The listing builds one solid part. Answer for the finished solid, in the listing's coordinates (mm). A direction names the side the tool comes from. Give positions to 0.01 mm unless a question says otherwise; leave off trailing zeros. Loops run counter-clockwise (first coordinate to the right, second up) from the corner with the lowest first, then second, coordinate; pieces in that order, holes last. Notation, with made-up numbers: M 13.5,-24 L 36.5,-24 A28 ccw 36.5,15 Z; hole C -3.5,-13.75 d8. An arc over 180 degrees is marked long. Return JSON: item names as keys, results as strings.
from build123d import *

# Parameters (mm, degrees)
SKETCH_1_W          = 54.664318292
SKETCH_1_H          = 5
SKETCH_1_R          = 1.5
EXTRUDE_1_DEPTH     = 5
SKETCH_2_W          = 59.460193076
SKETCH_2_H          = 2.500348526
EXTRUDE_2_DEPTH     = 23
SKETCH_5_R          = 16.5
CUT_EXTRUDE_1_DEPTH = 15
EXTRUDE_START       = 5
EXTRUDE_3_DEPTH     = 5
CHAMFER_1_SIZE      = 5
FILLET_6_R          = 10
FILLET_7_R          = 4
FILLET_8_R          = 5
FILLET_9_R          = 3


with BuildPart() as part:
    # 草图1 → 凸台-拉伸1 (new body)
    with BuildSketch(Plane(origin=(0, 0, 0), x_dir=(1, 0, 0), z_dir=(0, 1, 0))):
        with Locations((1.075531559, -8.61)):
            Rectangle(SKETCH_1_W, SKETCH_1_H)
        with Locations(Location((-10, -8.5, 0), (0, 0, 270))):
            Circle(SKETCH_1_R, mode=Mode.SUBTRACT)
        with Locations(Location((10, -8.5, 0), (0, 0, 90))):
            Circle(SKETCH_1_R, mode=Mode.SUBTRACT)
    extrude(amount=EXTRUDE_1_DEPTH)

    # 草图2 → 凸台-拉伸2 (add)
    with BuildSketch(Plane.XY.offset(11.11)):
        with Locations((0, 2.5)):
            Rectangle(SKETCH_2_W, SKETCH_2_H)
    extrude(amount=EXTRUDE_2_DEPTH)

    # 草图5 → 切除-拉伸1 (cut)
    with BuildSketch(Plane(origin=(0, 3.750174263, 0), x_dir=(1, 0, 0), z_dir=(0, 1, 0))):
        with Locations((-0.32, -44.994124541)):
            Circle(SKETCH_5_R)
    extrude(amount=-CUT_EXTRUDE_1_DEPTH, mode=Mode.SUBTRACT)

    # 草图7 → 凸台-拉伸3 (add)
    with BuildSketch(Plane(origin=(0, 3.750174263, 0), x_dir=(1, 0, 0), z_dir=(0, 1, 0)).offset(EXTRUDE_START)):
        with BuildLine():
            Line((29.730096538, -11.11), (28.407690705, -11.11))
            Line((28.407690705, -11.11), (-26.256627587, -11.11))
            Line((-26.256627587, -11.11), (-29.730096538, -11.11))
            Line((-29.730096538, -11.11), (-29.730096538, -34.11))
            Line((-29.730096538, -34.11), (-12.721041608, -34.11))
            ThreePointArc((-12.721041608, -34.11), (-0.32, -28.494124541), (12.081041608, -34.11))
            Line((12.081041608, -34.11), (29.730096538, -34.11))
            Line((29.730096538, -34.11), (29.730096538, -11.11))
        make_face()
    extrude(amount=-EXTRUDE_3_DEPTH)

    # 倒角1
    # the kernel refuses this chamfer: 5 mm, written as the material it takes off along each edge
    with BuildSketch(Plane(origin=(-42.588511478, 8.750174263, 11.11), x_dir=(0, -0.9996219169112968, -0.027495876610586317), z_dir=(1, 0, 0))) as chamfer_1_piece_1_section:
        Polygon((CHAMFER_1_SIZE * 0.999621916911, -CHAMFER_1_SIZE * 0.0274958766106), (-CHAMFER_1_SIZE * 0.0274958766106, -CHAMFER_1_SIZE * 0.999621916911), (0, 0), align=None)
    chamfer_1_piece_1 = extrude(amount=85.177022955, mode=Mode.PRIVATE)
    chamfer_1_piece_1 = split(chamfer_1_piece_1, bisect_by=Plane(origin=(-34.422569532, 5, 11.399404242), z_dir=(0, -1, 0)), keep=Keep.TOP, mode=Mode.PRIVATE)
    chamfer_1_piece_1 = split(chamfer_1_piece_1, bisect_by=Plane(origin=(-26.256627587, 4.506210637, 11.399404242), z_dir=(-1, 0, 0)), keep=Keep.TOP, mode=Mode.PRIVATE)
    add(chamfer_1_piece_1, mode=Mode.SUBTRACT)
    with BuildSketch(Plane(origin=(-42.588511478, 8.750174263, 11.11), x_dir=(0, -0.9996219169112968, -0.027495876610586317), z_dir=(1, 0, 0))) as chamfer_1_piece_2_section:
        Polygon((CHAMFER_1_SIZE * 0.999621916911, -CHAMFER_1_SIZE * 0.0274958766106), (-CHAMFER_1_SIZE * 0.0274958766106, -CHAMFER_1_SIZE * 0.999621916911), (0, 0), align=None)
    chamfer_1_piece_2 = extrude(amount=85.177022955, mode=Mode.PRIVATE)
    chamfer_1_piece_2 = split(chamfer_1_piece_2, bisect_by=Plane(origin=(-34.422569532, 5, 12.869772417), z_dir=(0, 1, 0)), keep=Keep.TOP, mode=Mode.PRIVATE)
    chamfer_1_piece_2 = split(chamfer_1_piece_2, bisect_by=Plane(origin=(-26.256627587, 7.312697929, 12.869772417), z_dir=(-1, 0, 0)), keep=Keep.TOP, mode=Mode.PRIVATE)
    add(chamfer_1_piece_2, mode=Mode.SUBTRACT)
    with BuildSketch(Plane(origin=(-42.588511478, 8.750174263, 11.11), x_dir=(0, -0.9996219169112968, -0.027495876610586317), z_dir=(1, 0, 0))) as chamfer_1_piece_3_section:
        Polygon((CHAMFER_1_SIZE * 0.999621916911, -CHAMFER_1_SIZE * 0.0274958766106), (-CHAMFER_1_SIZE * 0.0274958766106, -CHAMFER_1_SIZE * 0.999621916911), (0, 0), align=None)
    chamfer_1_piece_3 = extrude(amount=85.177022955, mode=Mode.PRIVATE)
    chamfer_1_piece_3 = split(chamfer_1_piece_3, bisect_by=Plane(origin=(1.075531559, 5, 12.869772417), z_dir=(0, 1, 0)), keep=Keep.TOP, mode=Mode.PRIVATE)
    chamfer_1_piece_3 = split(chamfer_1_piece_3, bisect_by=Plane(origin=(28.407690705, 7.312697929, 12.869772417), z_dir=(-1, 0, 0)), keep=Keep.TOP, mode=Mode.PRIVATE)
    chamfer_1_piece_3 = split(chamfer_1_piece_3, bisect_by=Plane(origin=(-26.256627587, 7.312697929, 12.869772417), z_dir=(1, 0, 0)), keep=Keep.TOP, mode=Mode.PRIVATE)
    add(chamfer_1_piece_3, mode=Mode.SUBTRACT)
    with BuildSketch(Plane(origin=(-42.588511478, 8.750174263, 11.11), x_dir=(0, -0.9996219169112968, -0.027495876610586317), z_dir=(1, 0, 0))) as chamfer_1_piece_4_section:
        Polygon((CHAMFER_1_SIZE * 0.999621916911, -CHAMFER_1_SIZE * 0.0274958766106), (-CHAMFER_1_SIZE * 0.0274958766106, -CHAMFER_1_SIZE * 0.999621916911), (0, 0), align=None)
    chamfer_1_piece_4 = extrude(amount=85.177022955, mode=Mode.PRIVATE)
    chamfer_1_piece_4 = split(chamfer_1_piece_4, bisect_by=Plane(origin=(35.498101091, 5, 11.399404242), z_dir=(0, -1, 0)), keep=Keep.TOP, mode=Mode.PRIVATE)
    chamfer_1_piece_4 = split(chamfer_1_piece_4, bisect_by=Plane(origin=(28.407690705, 4.506210637, 11.399404242), z_dir=(1, 0, 0)), keep=Keep.TOP, mode=Mode.PRIVATE)
    add(chamfer_1_piece_4, mode=Mode.SUBTRACT)
    with BuildSketch(Plane(origin=(-42.588511478, 8.750174263, 11.11), x_dir=(0, -0.9996219169112968, -0.027495876610586317), z_dir=(1, 0, 0))) as chamfer_1_piece_5_section:
        Polygon((CHAMFER_1_SIZE * 0.999621916911, -CHAMFER_1_SIZE * 0.0274958766106), (-CHAMFER_1_SIZE * 0.0274958766106, -CHAMFER_1_SIZE * 0.999621916911), (0, 0), align=None)
    chamfer_1_piece_5 = extrude(amount=85.177022955, mode=Mode.PRIVATE)
    chamfer_1_piece_5 = split(chamfer_1_piece_5, bisect_by=Plane(origin=(35.498101091, 5, 12.869772417), z_dir=(0, 1, 0)), keep=Keep.TOP, mode=Mode.PRIVATE)
    chamfer_1_piece_5 = split(chamfer_1_piece_5, bisect_by=Plane(origin=(28.407690705, 7.312697929, 12.869772417), z_dir=(1, 0, 0)), keep=Keep.TOP, mode=Mode.PRIVATE)
    add(chamfer_1_piece_5, mode=Mode.SUBTRACT)

    # 圆角6
    # the kernel refuses this fillet: 10 mm, written as the material it adds along each edge
    with BuildSketch(Plane(origin=(28.407690705, 1.249825737, 11.11), x_dir=(0, 0, 1), z_dir=(-1, 0, 0))) as fillet_6_piece_1:
        with BuildLine():
            CenterArc((4.840914208, -10), FILLET_6_R, 90, 28.952961909)
            Line((0, -1.249825737), (0, 0))
            Line((0, 0), (4.840914208, 0))
        make_face()
    extrude(amount=54.664318292)

    # 圆角7
    fillet_7_edges = [part.edges().sort_by_distance(p)[0] for p in [
        (0, 8.750174263, 16.11),
    ]]
    fillet(fillet_7_edges, radius=FILLET_7_R)

    # 圆角8
    fillet_8_edges = [part.edges().sort_by_distance(p)[0] for p in [
        (-12.721041608, 5, 34.11),
        (12.081041608, 5, 34.11),
    ]]
    fillet(fillet_8_edges, radius=FILLET_8_R)

    # 圆角9
    fillet_9_edges = [part.edges().sort_by_distance(p)[0] for p in [
        (-0.32, 1.249825737, 28.494124541),
        (21.949780623, 1.249825737, 34.11),
        (12.362521469, 1.249825737, 33.772076375),
        (-13.002521469, 1.249825737, 33.772076375),
        (-22.269780623, 1.249825737, 34.11),
    ]]
    fillet(fillet_9_edges, radius=FILLET_9_R)


solid = part.part
(1) The part is cut by section B-B (x = 15.5). Determine the outline of the cut face in (y, z).
Values follow:
{"outline": "M 0,6.11 L 5,6.11 L 5,12.36 L 7.58,14.94 A4 ccw 8.75,17.77 L 8.75,34.11 L 4.25,34.11 A3 ccw 1.25,31.11 L 1.25,15.95 A10 cw 0,11.11 Z"}
(2) Determine the mould class of faces 5 (the cylindrical face through (10.9, 2.5, 9.7)), 6 (the flat face through (1, 0, 9)), 7 (the flat face through (-29.73, 5, 22)) for opening direction X: released by +X, released by -X, zero draft, split by the parting line, or undercut.
Values follow:
{"face 5": "undercut", "face 6": "zero draft", "face 7": "released by -X"}
(3) The part is cut by section C-C (y = 6). Determine the outline of the cut face in (x, z), and give its area (3 significant figures).
Values follow:
{"outline": "M -29.73,13.36 L 29.73,13.36 L 29.73,34.11 L 14.17,34.11 A5 ccw 10.8,32.8 A16.5 cw -11.44,32.8 A5 ccw -14.81,34.11 L -29.73,34.11 Z", "area": "1,140 mm²"}
(4) Given pin 1 (6 mm diameter, centred on x = -4.5, z = 17.5, fed in from -Y); pin 2 (2 mm diameter, centred on x = -9.5, z = 20.5, fed in from -Y); pin 3 (2.5 mm diameter, centred on x = 10, z = 8.5, fed in from +Y); pin 4 (3 mm diameter, centred on x = -4, z = 9.5, fed in from +Y), each flat-ended and moving along its own axis, determine where each tip first touches the part or whether it passes through.
Values follow:
{"pin 1": "y = 1.14", "pin 2": "y = 1.25", "pin 3": "through", "pin 4": "y = 5"}
(5) The part is cut by section A-A (z = 8.5). Determine the outline of the cut face in (x, y), and give its area (3 significant figures).
Values follow:
{"outline": "M -26.26,0 L -11.5,0 L -11.5,5 L -26.26,5 Z; M -8.5,0 L 8.5,0 L 8.5,5 L -8.5,5 Z; M 11.5,0 L 28.41,0 L 28.41,5 L 11.5,5 Z", "area": "243 mm²"}
(6) The part is cut by section D-D (z = 18.75). Determine the outline of the cut face in (x, y).
Values follow:
{"outline": "M -29.73,1.25 L 29.73,1.25 L 29.73,8.75 L -29.73,8.75 Z"}
(7) Straight lines are drawn through the part: line 1 along X through (y, z) = (2.25, 8.5); line 2 along Y through (x, z) = (11.5, 22); line 3 along Y through (x, z) = (25, 8.5). For each, find the intervals that lie inside material, in ascending order.
Values follow:
{"line 1": "-26.26 to -11.5, -8.5 to 8.5, 11.5 to 28.41", "line 2": "1.25 to 8.75", "line 3": "0 to 5"}
(8) A tool of negligible diameter and unlimited length cuts with its end or side. For faces 1 (the cylindrical face through (-12.978, 6.468, 33.763)), 2 (the flat face through (-28, 3, 11.11)), 3 (the flat face through (29, 3, 11.11)), 4 (the flat face through (1, 5, 9)), from which of +Z, -Z, +X, -X, +Y, -Y can it reach the whole face along a straight path? Write none if from no direction.
Values follow:
{"face 1": "+Z, +Y, -Y", "face 2": "-Z, -X, +Y, -Y", "face 3": "-Z, +X, +Y, -Y", "face 4": "-Z, +X, -X, +Y"}
